The model under review builds one solid part; all positions refer to its coordinate system, in mm. Give positions to 0.01 mm unless a question says otherwise; leave off trailing zeros. Loops run counter-clockwise (first coordinate to the right, second up) from the corner with the lowest first, then second, coordinate; pieces in that order, holes last. Notation, with made-up numbers: (0, 73.5) - (50, 73.5) arc R21 cw to (50, 79.5) - close; hole circle Ø1 at (27.25, -27). An arc over 180 degrees is marked (long way). Return JSON: item names as keys, results as strings. Group by question number.
```python
from build123d import *

# Parameters (mm, degrees)
SKETCH1_R           = 78.359
SKETCH1_R_2         = 76.1746
BOSS_EXTRUDE1_DEPTH = 1016
SKETCH3_R           = 1.750000056
SKETCH3_R_2         = 1.0922
CUT_EXTRUDE1_DEPTH  = 1023.025570014
CIRPATTERN1_COUNT   = 4


with BuildPart() as part:
    # Sketch1 → Boss-Extrude1 (new body)
    with BuildSketch(Plane(origin=(0, 0, 0), x_dir=(1, 0, 0), z_dir=(0, 1, 0))):
        with Locations(Location((0, 0, 0), (0, 0, 270))):
            Circle(SKETCH1_R)
        with Locations(Location((0, 0, 0), (0, 0, 270))):
            Circle(SKETCH1_R_2, mode=Mode.SUBTRACT)
    extrude(amount=BOSS_EXTRUDE1_DEPTH)

    # Sketch3 → Cut-Extrude1 (cut, through all)
    with BuildSketch(Plane.XY):
        with Locations(Location((0, 558.8, 0), (0, 0, 90))):
            Circle(SKETCH3_R)
        with Locations(Location((0, 114.3, 0), (0, 0, 90))):
            Circle(SKETCH3_R_2)
        with Locations(Location((0, 901.7, 0), (0, 0, 90))):
            Circle(SKETCH3_R_2)
    cut_extrude1 = extrude(amount=-CUT_EXTRUDE1_DEPTH, mode=Mode.SUBTRACT)

    # CirPattern1: Cut-Extrude1 ×4 about axis
    cirpattern1_axis = Axis((0, 1016, 0), (0, -1, 0))
    for i in range(1, CIRPATTERN1_COUNT):
        add(cut_extrude1.rotate(cirpattern1_axis, i * 360 / CIRPATTERN1_COUNT), mode=Mode.SUBTRACT)


solid = part.part
```
1) We need section A-A, the plane z = 32. Write out the cut boundary in (x, y).
2) For pin 1 Ø3 at (x, y) = (59.5, 308) entering from +Z; pin 2 Ø8 at (x, y) = (44, 439) entering from -Z; pin 3 Ø6 at (x, y) = (-14, 313) entering from -Z, all flat-tipped, find the tip position at first contact; note any pin that passes through.
3) Draft analysis for pull direction Z (two halves, no side actions). For faces 1 (the face through (76, 0, -12)), 2 (the face through (22.881, 500.888, 72.657)), 3 (the face through (23.54, 500.89, 74.74)), state which applies: +Z half, -Z half, draft (parallel to the pull), parting line (faces both ways), or undercut.
4) We need section C-C, the plane y = 703. Write out the cut boundary in (x, z), plus the area to 3 significant figures.
5) To check wall thickness, follow line 1 (Z direction, x = 4, y = 777); line 2 (X direction, y = 322.5, z = 0); line 3 (X direction, y = 912, z = -2.5). State the ranges of each line that lie inside material, in increasing order.
6) We need section B-B, the plane x = 40. Write out the cut boundary in (y, z), plus the area to 3 significant figures.
Findings:
{
 "1": {"outline": "(-71.53, 0) - (-69.13, 0) - (-69.13, 1016) - (-71.53, 1016) - close; (69.13, 0) - (71.53, 0) - (71.53, 1016) - (69.13, 1016) - close"},
 "2": {"pin 1": "stops at z = 52.69", "pin 2": "stops at z = -67.38", "pin 3": "stops at z = -77.58"},
 "3": {"face 1": "draft", "face 2": "undercut", "face 3": "parting line"},
 "4": {"outline": "circle Ø156.72 at (0, 0); hole circle Ø152.35 at (0, 0)", "area": "1,060 mm^2"},
 "5": {"line 1": "z = -78.26 to -76.07, 76.07 to 78.26", "line 2": "x = -78.36 to -76.17, 76.17 to 78.36", "line 3": "x = -78.32 to -76.13, 76.13 to 78.32"},
 "6": {"outline": "(0, -67.38) - (1016, -67.38) - (1016, -64.83) - (0, -64.83) - close; (0, 64.83) - (1016, 64.83) - (1016, 67.38) - (0, 67.38) - close", "area": "5,190 mm^2"}
}
